from build123d import *

# Parameters (mm, degrees)
SKETCH2_R                  = 16
SKETCH2_R_2                = 11
BOSS_EXTRUDE1_DEPTH        = 7
M3X0_5_TAPPED_HOLE1_REACH  = 39.437
M3X0_5_TAPPED_HOLE1_BORE_R = 1.25
M3X0_5_TAPPED_HOLE2_D      = 2.5
M3X0_5_TAPPED_HOLE2_DEPTH  = 3.248924226
M3X0_5_TAPPED_HOLE2_TIP    = 0.751075774


with BuildPart() as part:
    # Sketch2 → Boss-Extrude1 (new body)
    with BuildSketch(Plane(origin=(0, 0, 0), x_dir=(1, 0, 0), z_dir=(0, 1, 0))):
        with Locations(Location((0, 0, 0), (0, 0, 270))):
            Circle(SKETCH2_R)
        with Locations(Location((0, 0, 0), (0, 0, 270))):
            Circle(SKETCH2_R_2, mode=Mode.SUBTRACT)
    extrude(amount=BOSS_EXTRUDE1_DEPTH)

    # M3x0.5 Tapped Hole1 bore (on position points) → M3x0.5 Tapped Hole1 (cut, up to next)
    with BuildSketch(Plane(origin=(-15.520289871, 3.526588003, -3.888521866), x_dir=(0.243032616649, 0, -0.970018116967), z_dir=(-0.970018116967, 0, -0.243032616649)), mode=Mode.PRIVATE) as m3x0_5_tapped_hole1_sk1:
        Circle(M3X0_5_TAPPED_HOLE1_BORE_R)
    m3x0_5_tapped_hole1_tool1 = extrude(m3x0_5_tapped_hole1_sk1.sketch, amount=-M3X0_5_TAPPED_HOLE1_REACH, mode=Mode.PRIVATE) & part.part
    add(m3x0_5_tapped_hole1_tool1.solids().sort_by_distance((-15.52029, 3.526588, -3.888522))[0], mode=Mode.SUBTRACT)

    # M3x0.5 Tapped Hole2
    with Locations(Plane(origin=(15.411877549, 3.498112916, 4.298142669), x_dir=(-0.268633916838, 0, 0.963242346829), z_dir=(0.963242346829, 0, 0.268633916838))):
        with Locations((0, 0)):
            Hole(M3X0_5_TAPPED_HOLE2_D / 2, depth=M3X0_5_TAPPED_HOLE2_DEPTH)
            with Locations((0, 0, -(M3X0_5_TAPPED_HOLE2_DEPTH + M3X0_5_TAPPED_HOLE2_TIP / 2))):  # 118° drill point
                Cone(0, M3X0_5_TAPPED_HOLE2_D / 2, M3X0_5_TAPPED_HOLE2_TIP, mode=Mode.SUBTRACT)


solid = part.part
Build history of the part. All positions in model axes, mm. A direction names the side the tool comes from. Give positions to 0.01 mm unless a question says otherwise; leave off trailing zeros. Order: outer loops, then holes, each group sorted by start corner. A loop starts at its lowest first (then second) coordinate and runs counter-clockwise, first axis right, second up. Notation, with made-up numbers: M 41,-33.5 L 83,-33.5 A12 ccw 83,-23.5 Z; hole C -23,51 d10. An arc over 180 degrees is marked long. Put each result on its own line as item: value.
Item 1: Drop flat-ended pins along their axis: pin 1 Ø4 at (x, y) = (12.5, 0.5) entering from +Z; pin 2 Ø4 at (x, y) = (-4.5, 2.5) entering from -Z; pin 3 Ø4 at (y, z) = (3.5, 1.5) entering from -X; pin 4 Ø1 at (y, z) = (3.5, 5) entering from -X. Give the stop position or say it passes through.
Results are:
pin 1: z = 12.07
pin 2: z = -15.8
pin 3: x = -16
pin 4: x = -15.35
Item 2: Which spindle directions (+Z, -Z, +X, -X, +Y, -Y) get a long thin tool onto all of the face, cutting with end or side? Do faces 1 (the face through (11.63, 3.58, 3.45)), 2 (the face through (10.906, 3.451, -1.432)). Say none if no direction does.
Results are:
face 1: none
face 2: +Y, -Y
Item 3: Cut at C-C on y = 6. Write the cut outline in (x, z).
Results are:
outline: C 0,0 d32; hole C 0,0 d22
Item 4: Cut at A-A on x = 0. Write the cut outline in (y, z).
Results are:
outline: M 0,-16 L 7,-16 L 7,-11 L 0,-11 Z; M 0,11 L 7,11 L 7,16 L 0,16 Z
Item 5: Cut at B-B on z = 0. Write the cut outline in (x, y), then the cut area to 3 significant figures.
Results are:
outline: M -16,0 L -11,0 L -11,7 L -16,7 Z; M 11,0 L 16,0 L 16,7 L 11,7 Z
area: 70.0 mm2
Item 6: Wall check: probe 1 along X at (y, z) = (3, 0); probe 2 along Z at (x, y) = (-1.5, 2.75); probe 3 along X at (y, z) = (1.25, -9). Give the ranges that are in metal, low to high.
Results are:
probe 1: -16 to -11, 11 to 16
probe 2: -15.93 to -10.9, 10.9 to 15.93
probe 3: -13.23 to -6.32, 6.32 to 13.23
Item 7: Pull direction Z, two halves, no side cores. Call faces 3 (the face through (-12.8, 4, -4.4)), 4 (the face through (13.78, 2.26, 4.01)), 5 (the face through (15.864, 3.451, -2.083)), 6 (the face through (11, 7, 3)): +Z half, -Z half, draft (parallel to the pull), parting line (faces both ways), or undercut.
Results are:
face 3: undercut
face 4: undercut
face 5: parting line
face 6: draft
Item 8: Cut at D-D on z = -3.5. Count the separate pieces of the cut face and the enclosed holes in it, then the cut area to 3 significant figures.
Results are:
separate pieces: 3
enclosed holes: 0
area: 60.4 mm2
